For this review, take the finished solid that the model builds, in its own axes (mm). Face numbers are marked on the shaded views. A direction names the side the tool comes from. Give positions to 0.01 mm unless a question says otherwise; leave off trailing zeros. Write each loop counter-clockwise with the first axis right and the second up, starting at its lowest first coordinate (ties: lowest second). Pieces come first, ordered by that corner, then holes.
1) Wall thickness on line 1 along Y through (x, z) = (-14, 48); line 2 along Z through (x, y) = (-9.5, 7); line 3 along Z through (x, y) = (4, -12.5): over which ranges is each line inside the solid? List them lowest first.
2) Draft analysis for pull direction Z (two halves, no side actions). For the marked faces 1, 2, 3 and 4, state which applies: pulls with the +Z half, pulls with the -Z half, needs draft (parallel to the pull), parting line crosses it, or undercut.
3) We need section B-B on y = 0. Give the boundary of the cut face in (x, z).
4) We need section C-C on x = -10. Give the boundary of the cut face in (y, z), and give its area (3 significant figures).
5) We need section A-A on z = 47.5. Give the boundary of the cut face in (x, y).
6) Machinability: for the marked faces 5, 6 and 7, which of the approach directions +Z, -Z, +X, -X, +Y, -Y give a long, thin tool a straight path to every point of the face, cutting with its end or side? Answer none if there is none.
7) We need section D-D on z = 35. Give the boundary of the cut face in (x, y).
8) For P1, Ø3.5, axis at y = -9, z = 66, coming from the -X side; P2, Ø1.9, axis at x = 14, y = -14, coming from the -Z side; P3, Ø4.5, axis at y = -2.5, z = 35, coming from the +X side; P4, Ø4, axis at y = -9.5, z = 43, coming from the -X side, all flat-tipped, find the tip position at first contact; note any pin that passes through.
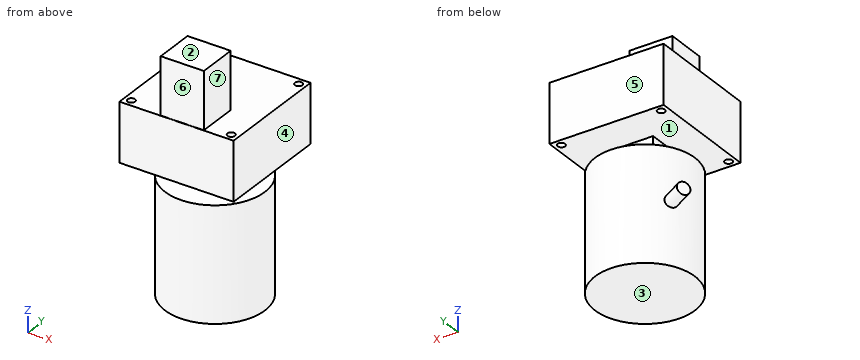
from build123d import *

# Parameters (mm, degrees)
SKETCH_1_R          = 14
EXTRUDE_1_DEPTH     = 32
SKETCH_2_W          = 12
SKETCH_2_H          = 11
EXTRUDE_2_DEPTH     = 5.8
SKETCH_3_W          = 32
SKETCH_3_H          = 32
EXTRUDE_3_DEPTH     = 16.5
SKETCH_4_W          = 12.1
SKETCH_4_H          = 11.16
EXTRUDE_4_DEPTH     = 16
SKETCH_5_R          = 1.05
CUT_EXTRUDE_1_DEPTH = 16.5
EXTRUDE_START       = -21.86
SKETCH_6_R          = 1.75
EXTRUDE_6_DEPTH     = 20.5


with BuildPart() as part:
    # 草图1 → 凸台-拉伸1 (new body)
    with BuildSketch(Plane.XY):
        Circle(SKETCH_1_R)
    extrude(amount=EXTRUDE_1_DEPTH)

    # 草图2 → 凸台-拉伸2 (add)
    with BuildSketch(Plane.XY.offset(32)):
        Rectangle(SKETCH_2_W, SKETCH_2_H)
    extrude(amount=EXTRUDE_2_DEPTH)

    # 草图3 → 凸台-拉伸3 (add)
    with BuildSketch(Plane.XY.offset(37.8)):
        Rectangle(SKETCH_3_W, SKETCH_3_H)
    extrude(amount=EXTRUDE_3_DEPTH)

    # 草图4 → 凸台-拉伸4 (add)
    with BuildSketch(Plane.XY.offset(54.3)):
        with Locations((1.55, -10.32)):
            Rectangle(SKETCH_4_W, SKETCH_4_H)
    extrude(amount=EXTRUDE_4_DEPTH)

    # 草图5 → 切除-拉伸1 (cut)
    with BuildSketch(Plane.XY.offset(54.3)):
        with Locations((-14, 14)):
            Circle(SKETCH_5_R)
        with Locations((14, 14)):
            Circle(SKETCH_5_R)
        with Locations((-14, -14)):
            Circle(SKETCH_5_R)
        with Locations((14, -14)):
            Circle(SKETCH_5_R)
    extrude(amount=-CUT_EXTRUDE_1_DEPTH, mode=Mode.SUBTRACT)

    # 草图6 → 凸台-拉伸6 (add)
    with BuildSketch(Plane(origin=(-18.92820323, 10.92820323, 0), x_dir=(0, 0, -1), z_dir=(-0.8660254037844398, 0.499999999999998, 0)).offset(EXTRUDE_START)):
        with Locations(Location((-17.5, 0, 0), (0, 0, 270))):
            Circle(SKETCH_6_R)
    extrude(amount=EXTRUDE_6_DEPTH)


solid = part.part
Results list:
1. line 1: y = -16 to -15.05, -12.95 to 12.95, 15.05 to 16
1. line 2: z = 0 to 32, 37.8 to 54.3
1. line 3: z = 0 to 32, 37.8 to 70.3
2. face 1: undercut
2. face 2: pulls with the +Z half
2. face 3: pulls with the -Z half
2. face 4: needs draft
3. outline: (-16, 37.8) - (-6, 37.8) - (-6, 32) - (-14, 32) - (-14, 0) - (14, 0) - (14, 32) - (6, 32) - (6, 37.8) - (16, 37.8) - (16, 54.3) - (-16, 54.3) - close
4. outline: (-16, 37.8) - (16, 37.8) - (16, 54.3) - (-16, 54.3) - close; (-9.8, 0) - (9.8, 0) - (9.8, 32) - (-9.8, 32) - close
4. area: 1,160 mm2
5. outline: (-16, -16) - (16, -16) - (16, 16) - (-16, 16) - close; hole circle Ø2.1 at (-14, -14); hole circle Ø2.1 at (-14, 14); hole circle Ø2.1 at (14, -14); hole circle Ø2.1 at (14, 14)
6. face 5: +Z, -Z, +X, -X, +Y
6. face 6: +Z, +X, -X, -Y
6. face 7: +Z, +X, +Y, -Y
7. outline: (-6, -5.5) - (6, -5.5) - (6, 5.5) - (-6, 5.5) - close
8. P1: stops at x = -4.5
8. P2: passes through
8. P3: stops at x = 6
8. P4: stops at x = -16
